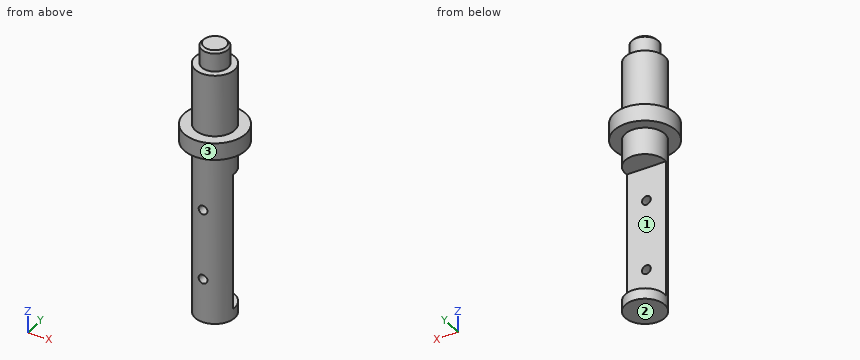
from build123d import *

# Parameters (mm, degrees)
CUT_EXTRUDE1_DEPTH      = 205.420962722
CUT_EXTRUDE1_DEPTH_BACK = 205.420962722
SKETCH2_W               = 193.8
SKETCH2_H               = 37.910107369
CUT_EXTRUDE2_DEPTH      = 205.420962722
CUT_EXTRUDE2_DEPTH_BACK = 205.420962722
SKETCH3_R               = 6.25
CHAMFER1_SIZE           = 3


with BuildPart() as part:
    # Sketch1 → Revolve1 (revolve)
    with BuildSketch(Plane(origin=(0, 0, 0), x_dir=(0, 0, -1), z_dir=(1, 0, 0)), mode=Mode.PRIVATE) as revolve1_sk:
        Polygon((192.6, 0), (192.6, 28), (-54.5, 28), (-54.5, 43.6), (-78.5, 43.6), (-78.5, 28), (-166, 28), (-166, 18.75), (-194.9, 18.75), (-194.9, 0), align=None)
    revolve(revolve1_sk.sketch.rotate(Axis((0, 0, 76.367145791), (0, 0, -1)), 90), axis=Axis((0, 0, 76.367145791), (0, 0, -1)))

    # Sketch2 → Cut-Extrude1 (cut, two sides: drawn at the far end of the back side and taken through both)
    with BuildSketch(Plane(origin=(0, 0, 0), x_dir=(0, 0, -1), z_dir=(1, 0, 0)).offset(-CUT_EXTRUDE1_DEPTH_BACK)):
        with Locations((80.6, 15.855053684)):
            Rectangle(SKETCH2_W, SKETCH2_H)
    extrude(amount=CUT_EXTRUDE1_DEPTH + CUT_EXTRUDE1_DEPTH_BACK, mode=Mode.SUBTRACT)

    # Sketch3 → Cut-Extrude2 (cut, two sides: drawn at the far end of the back side and taken through both)
    with BuildSketch(Plane(origin=(0, 0, 0), x_dir=(1, 0, 0), z_dir=(0, 1, 0)).offset(-CUT_EXTRUDE2_DEPTH_BACK)):
        with Locations(Location((0, 30.6, 0), (0, 0, 270))):
            Circle(SKETCH3_R)
        with Locations(Location((0, 130.6, 0), (0, 0, 270))):
            Circle(SKETCH3_R)
    extrude(amount=CUT_EXTRUDE2_DEPTH + CUT_EXTRUDE2_DEPTH_BACK, mode=Mode.SUBTRACT)

    # Chamfer1
    chamfer1_edges = [part.edges().sort_by_distance(p)[0] for p in [
        (-18.75, 0, 194.9),
    ]]
    chamfer(chamfer1_edges, length=CHAMFER1_SIZE)


solid = part.part
Can you work these out from the model? Positions are in its coordinate system, mm. Face numbers are marked on the shaded views. Round coordinates to 2 decimals unless told otherwise and drop trailing zeros. Write each loop counter-clockwise with the first axis right and the second up, starting at its lowest first coordinate (ties: lowest second). Pieces come first, ordered by that corner, then holes. Notation, with made-up numbers: (54, 81) -> (80, 81) arc R21 cw to (80, 100) -> close; hole circle Ø3 at (48.5, 31.25). An arc over 180 degrees is marked (long way). Use one line per item in the form item = value. Start each with the question number.
Q1. Imagine slicing it at D-D (y = -33). Please give me the cut outline in (x, z), then the cut area to 3 significant figures.
Q2. Imagine slicing it at C-C (z = -84.5). Please give me the cut outline in (x, y), then the cut area to 3 significant figures.
Q3. Imagine slicing it at A-A (x = 0). Count the separate pieces of the cut face and the enclosed holes in it, then the cut area to 3 significant figures.
Q4. We'd pull the mould along Z, two halves only. Please class the marked faces 1, 2 and 3: +Z half, -Z half, draft (parallel to the pull), parting line (faces both ways), or undercut.
Q5. Imagine slicing it at B-B (z = -130.6). Please give me the cut outline in (x, y), then the cut area to 3 significant figures.
Q6. If I drill on probe 1 along Z at (x, y) = (0, -22.5); probe 2 along Z at (x, y) = (0, -11.75); probe 3 along Z at (x, y) = (1, 1.5), over which ranges is the centre line in solid material (lowest first)? Write a range as [from, to].
Q7. I'm going to push flat-ended pins straight in: P1, Ø8, axis at x = 22, y = -29.5, coming from the -Z side; P2, Ø4, axis at x = 20.5, z = 33.5, coming from the -Y side; P3, Ø20, axis at x = 0, z = -130.6, coming from the +Y side. Where does each tip first touch, or does it pass through?
Worked out:
q1.outline = (-28.49, 54.5) -> (28.49, 54.5) -> (28.49, 78.5) -> (-28.49, 78.5) -> close
q1.area = 1,370 mm^2
q2.outline = (-27.83, -3.1) arc R28 ccw to (27.83, -3.1) -> close
q2.area = 1,060 mm^2
q3.separate_pieces = 3
q3.enclosed_holes = 0
q3.area = 15,300 mm^2
q4.face_1 = undercut
q4.face_2 = -Z half
q4.face_3 = draft
q5.outline = (-27.83, -3.1) arc R28 ccw to (-6.25, -27.29) -> (-6.25, -3.1) -> close; (6.25, -27.29) arc R28 ccw to (27.83, -3.1) -> (6.25, -3.1) -> close
q5.area = 750 mm^2
q6.probe_1 = [-192.6, -136.85], [-124.35, -36.85], [-24.35, 166]
q6.probe_2 = [-192.6, -136.85], [-124.35, -36.85], [-24.35, 194.9]
q6.probe_3 = [-192.6, -177.5], [16.3, 194.9]
q7.P1 = 54.5
q7.P2 = -21.02
q7.P3 = -3.1
